Autodesk Inventor part; units mm, degrees
ref_plane "EPHUB_XY" through (0, 5, 0) normal (0, 1, 0) x (1, 0, 0)
ref_plane "EPHUB_YZ" through (0, 5, 0) normal (1, 0, 0) x (0, 0, -1)
ref_plane "EPHUB_ZX" through (0, 5, 0) normal (0, 0, -1) x (0, 1, 0)
sketch "Skizze_1" plane through (0, 0, 0) normal (0, 0, 1) x (1, 0, 0)
  line L0 (0, 40) -> (6.773, 40)
  line L1 (6.773, 40) -> (8, 38.773)
  line L2 (8, 38.773) -> (8, 5)
  line L3 (8, 5) -> (20, 5)
  line L4 (20, 5) -> (20, 0)
  line L5 (20, 0) -> (18, 0)
  line L6 (18, 0) -> (18, -93.0264)
  line L7 (18, -93.0264) -> (0, -93.0264)
  line L8 (0, -93.0264) -> (0, 40)
revolve "Revolution1" add sketch "Skizze_1" angle 360 about axis through (0, -93.0264, 0) along (0, -1, 0)
thread "Thread1"
sketch "Skizze_2" plane through (0, 40, 0) normal (0, 1, 0) x (1, 0, 0)
  line L0 (-4, -2.3094) -> (0, -4.6188)
  line L1 (0, -4.6188) -> (4, -2.3094)
  line L2 (4, -2.3094) -> (4, 2.3094)
  line L3 (4, 2.3094) -> (0, 4.6188)
  line L4 (0, 4.6188) -> (-4, 2.3094)
  line L5 (-4, 2.3094) -> (-4, -2.3094)
extrude "Extrusion1" cut sketch "Skizze_2" against normal blind 12.4
ref_plane "EPHUB_XY" through (0, 5, 0) normal (0, 1, 0) x (1, 0, 0)
ref_plane "EPHUB_YZ" through (0, 5, 0) normal (1, 0, 0) x (0, 0, -1)
ref_plane "EPHUB_ZX" through (0, 5, 0) normal (0, 0, -1) x (0, 1, 0)
ref_plane "EPZAPFEN_XY" through (0, 0, 0) normal (0, 1, 0) x (1, 0, 0)
ref_plane "EPZAPFEN_YZ" through (0, 0, 0) normal (1, 0, 0) x (0, 0, -1)
ref_plane "EPZAPFEN_ZX" through (0, 0, 0) normal (0, 0, -1) x (0, 1, 0)
sketch "Boceto3" plane through (0, 5, 0) normal (0, 1, 0) x (1, 0, 0)
  point P0 (0, 0)
sketch "Boceto4" plane through (0, 40, 0) normal (0, 1, 0) x (1, 0, 0)
  circle A0 centre (0, 0) radius 8
  dimension "d7" = 16
extrude "Extrusión2" cut sketch "Boceto4" against normal blind 20
properties part number "LZ80_Zapfen"
Verification items for the finished model (mm, model axes). A direction names the side the tool comes from. Coordinates: 2 decimals unless noted, no trailing zeros. Order: outer loops, then holes, each group sorted by start corner. A loop starts at its lowest first (then second) coordinate and runs counter-clockwise, first axis right, second up.
Item 1: Material ranges on L1, parallel to Y at x = -14.5, z = -10; L2, parallel to Y at x = 17.5, z = -5; L3, parallel to Z at x = -6.5, y = -53.5, recorded low to high.
Filled in:
L1: y = -93.03 to 5
L2: y = 0 to 5
L3: z = -16.79 to 16.79
Item 2: Section check D-D, the plane z = 0. Enter the section's corners in (x, y).
Filled in:
outline: (-20, 0) - (-18, 0) - (-18, -93.03) - (18, -93.03) - (18, 0) - (20, 0) - (20, 5) - (8, 5) - (8, 20) - (-8, 20) - (-8, 5) - (-20, 5) - close
Item 3: Section check B-B, the plane z = -11.5. Enter the section's corners in (x, y).
Filled in:
outline: (-16.36, 0) - (-13.85, 0) - (-13.85, -93.03) - (13.85, -93.03) - (13.85, 0) - (16.36, 0) - (16.36, 5) - (-16.36, 5) - close
Item 4: Section check C-C, the plane y = -83. Enter the section's corners in (x, z), then the cut area to 3 significant figures.
Filled in:
outline: circle Ø36 at (0, 0)
area: 1,020 mm2
Item 5: Access from +Z, -Z, +X, -X, +Y, -Y to the whole of each face (thin tool, end or side, straight path). Record for faces 1 (the face through (-4.336, 2.465, -19.524)), 2 (the face through (-18, 0, 3)), 3 (the face through (9, 5, 0)).
Filled in:
face 1: +Y, -Y
face 2: -Y
face 3: +Y
Item 6: Section check A-A, the plane x = 0. Enter the section's corners in (y, z).
Filled in:
outline: (-93.03, -18) - (0, -18) - (0, -20) - (5, -20) - (5, -8) - (20, -8) - (20, 8) - (5, 8) - (5, 20) - (0, 20) - (0, 18) - (-93.03, 18) - close
Item 7: Depth check by flat-ended pin: pin 1 (4 mm diameter, centred on x = 14, z = -8, fed in from +Y); pin 2 (5 mm diameter, centred on y = -52, z = -15.5, fed in from -X); pin 3 (2 mm diameter, centred on y = 6.5, z = -14, fed in from +X) (1 decimal); pin 4 (2 mm diameter, centred on x = -1.5, y = -72, fed in from +Z). Enter the tip coordinate at first touch or a pass-through.
Filled in:
pin 1: stops at y = 5
pin 2: stops at x = -12.45
pin 3: passes through
pin 4: stops at z = 17.99
